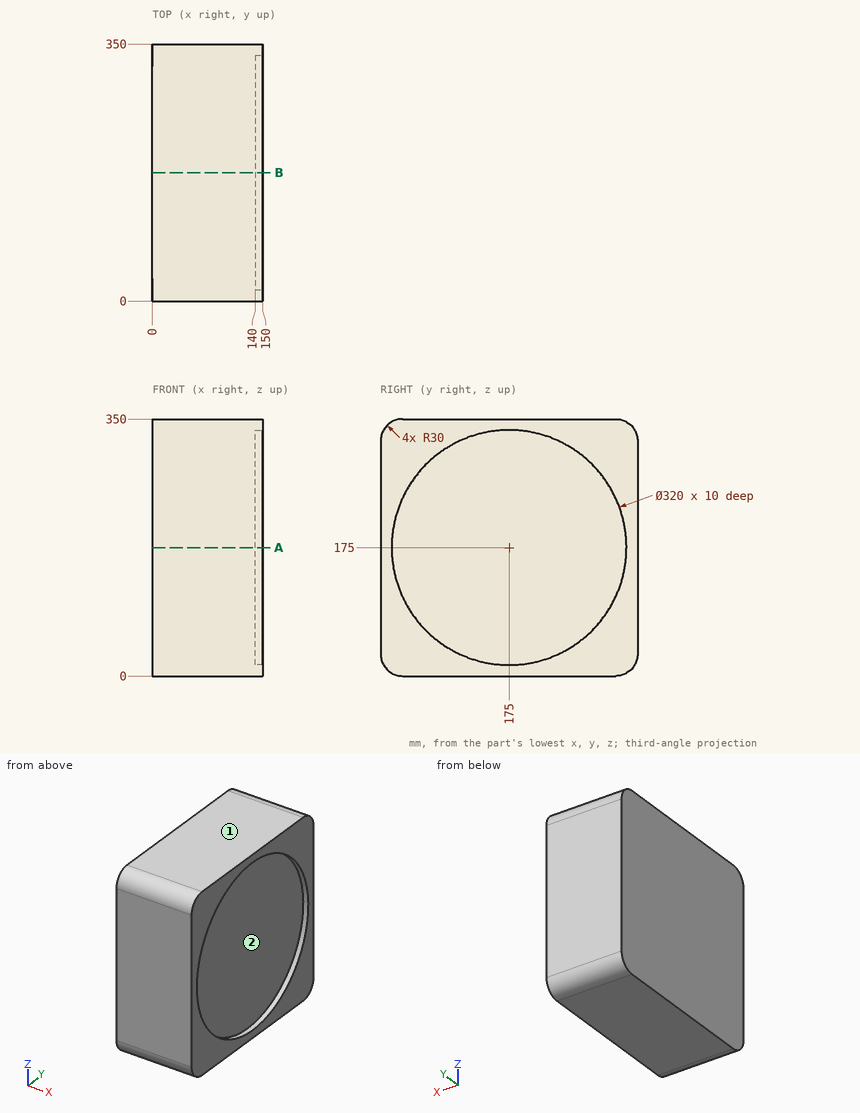
For this review, use the dimensioned drawing (mm, ordinates from the lowest corner) and the shaded views. A direction names the side the tool comes from. Give positions to 0.01 mm unless a question says otherwise; leave off trailing zeros. Loops run counter-clockwise (first coordinate to the right, second up) from the corner with the lowest first, then second, coordinate; pieces in that order, holes last. Notation, with made-up numbers: (-31, -26.75) -> (-10, -26.75) arc R26 ccw to (-10, 8.25) -> close; hole circle Ø10 at (-9.5, -8.75). An arc over 180 degrees is marked (long way). One line per question, with ' | ' between items. Start each with the question number.
(1) For the marked faces 1 and 2, list the 3-axis set-ups (+Z, -Z, +X, -X, +Y, -Y) from which the entire face can be reached by the end or side of a thin tool; tool diameter is ignored.
(2) We need section A-A (z = 175). State the section outline as (x, y) points, and give its area (3 significant figures).
(3) For line 1 (Y direction, x = 147, z = 175); line 2 (X direction, y = 158, z = 324.5); line 3 (Z direction, x = 22, y = 323), list the stretches that pass through material, from the lowest coordinate up.
(4) Insertion check: P1, Ø4, axis at y = 295, z = 167.5, coming from the +X side. The pin has a flat end and moves straight along its axis. Give the tip position at first contact, or say it passes through.
The answers:
1) face 1: +Z, +X, -X, +Y, -Y | face 2: +X
2) outline: (0, 0) -> (150, 0) -> (150, 15) -> (140, 15) -> (140, 335) -> (150, 335) -> (150, 350) -> (0, 350) -> close | area: 49,300 mm^2
3) line 1: y = 0 to 15, 335 to 350 | line 2: x = 0 to 140 | line 3: z = 0.15 to 349.85
4) P1: stops at x = 140
